Autodesk Inventor part; units mm, degrees
ref_plane "YZ Plane" through (0, 0, 0) normal (1, 0, 0) x (0, 1, 0)
ref_plane "XZ Plane" through (0, 0, 0) normal (0, 1, 0) x (-1, 0, 0)
ref_plane "XY Plane" through (0, 0, 0) normal (0, 0, 1) x (1, 0, 0)
sketch "Sketch1" plane through (0, 0, 0) normal (0, 0, 1) x (1, 0, 0)
  circle A0 centre (0, 0) radius 18.0213
  circle A1 centre (0, 0) radius 4
  circle A2 centre (0, 0) radius 11.0236
  circle A3 centre (0, 0) radius 6.35
  dimension "d0" = 36.0426
  dimension "d1" = 8
  dimension "d2" = 22.0472
  dimension "d9" = 12.7
extrude "Extrusion1" add sketch "Sketch1" along normal blind 107.95 contours A0 | A1 | A2 | A3
extrude "Extrusion2" add sketch "Sketch1" against normal blind 2.0701 contours A2 | A3
extrude "Extrusion3" add sketch "Sketch1" against normal blind 19.9009 contours A1
extrude "Extrusion4" add sketch "Sketch1" along normal blind 111.2012 contours A1 | A3
properties part number "DriveMotor"
Source: CAD feature listing. Evaluate the final solid. Frame: model axes, mm. A direction names the side the tool comes from. Give positions to 0.01 mm unless a question says otherwise; leave off trailing zeros. Write each loop counter-clockwise with the first axis right and the second up, starting at its lowest first coordinate (ties: lowest second). Pieces come first, ordered by that corner, then holes. Notation, with made-up numbers: M 9.5,24.5 L 64.5,24.5 A31 ccw 64.5,51.5 Z; hole C 83,46.5 d1. An arc over 180 degrees is marked long. Return JSON: item names as keys, results as strings. Group by question number.
1) Cut plane B-B, the plane x = 9. Output: boundary loops of the cut face in (y, z).
2) First-contact query: pin 1 Ø5 at (x, z) = (-10, 29.5) entering from -Y; pin 2 Ø1.5 at (x, z) = (0.5, 7.5) entering from -Y; pin 3 Ø1 at (x, z) = (2, 18.5) entering from +Y. Flat tips, straight axial feed; report the tip coordinate or a pass-through.
3) Ray query, L1, parallel to Z at x = 6, y = -16; L2, parallel to Z at x = -6, y = -9; L3, parallel to X at y = -1, z = 46. Return the intervals inside material, ascending.
4) Cut plane C-C, the plane z = 48.5. Output: boundary loops of the cut face in (x, y), then the cut area to 3 significant figures.
5) Set-up query: faces 1 (the face through (-1.38, 6.2, 109.55)), 2 (the face through (5, 0, -2.07)), 3 (the face through (0, 0, -19.901)). Return all of +Z, -Z, +X, -X, +Y, -Y with unobstructed straight access to the full face (end or side cutting, diameter ignored); none if empty.
6) Cut plane A-A, the plane y = 0. Output: boundary loops of the cut face in (x, z), then the cut area to 3 significant figures.
7) Cut plane D-D, the plane x = -1. Output: boundary loops of the cut face in (y, z), then the cut area to 3 significant figures.
Data:
{
 "1": {"outline": "M -15.61,0 L -6.37,0 L -6.37,-2.07 L 6.37,-2.07 L 6.37,0 L 15.61,0 L 15.61,107.95 L -15.61,107.95 Z"},
 "2": {"pin 1": "stops at y = -16.39", "pin 2": "stops at y = -18.02", "pin 3": "stops at y = 17.96"},
 "3": {"L1": "z = 0 to 107.95", "L2": "z = -2.07 to 107.95", "L3": "x = -17.99 to 17.99"},
 "4": {"outline": "C 0,0 d36.04", "area": "1,020 mm²"},
 "5": {"face 1": "+Z", "face 2": "-Z", "face 3": "-Z, +X, -X, +Y, -Y"},
 "6": {"outline": "M -18.02,0 L -11.02,0 L -11.02,-2.07 L -4,-2.07 L -4,-19.9 L 4,-19.9 L 4,-2.07 L 11.02,-2.07 L 11.02,0 L 18.02,0 L 18.02,107.95 L 6.35,107.95 L 6.35,111.2 L -6.35,111.2 L -6.35,107.95 L -18.02,107.95 Z", "area": "4,120 mm²"},
 "7": {"outline": "M -17.99,0 L -10.98,0 L -10.98,-2.07 L -3.87,-2.07 L -3.87,-19.9 L 3.87,-19.9 L 3.87,-2.07 L 10.98,-2.07 L 10.98,0 L 17.99,0 L 17.99,107.95 L 6.27,107.95 L 6.27,111.2 L -6.27,111.2 L -6.27,107.95 L -17.99,107.95 Z", "area": "4,110 mm²"}
}
